Can you work these out from the model? Positions are in its coordinate system, mm. Face numbers are marked on the shaded views. A direction names the side the tool comes from. Round coordinates to 2 decimals unless told otherwise and drop trailing zeros. Order: outer loops, then holes, each group sorted by start corner. A loop starts at its lowest first (then second) coordinate and runs counter-clockwise, first axis right, second up. Notation, with made-up numbers: (3.5, -17) -> (28.5, -17) arc R28 ccw to (28.5, 10) -> close; hole circle Ø3 at (43.5, 49). An arc over 180 degrees is marked (long way). One line per item, written item: value.
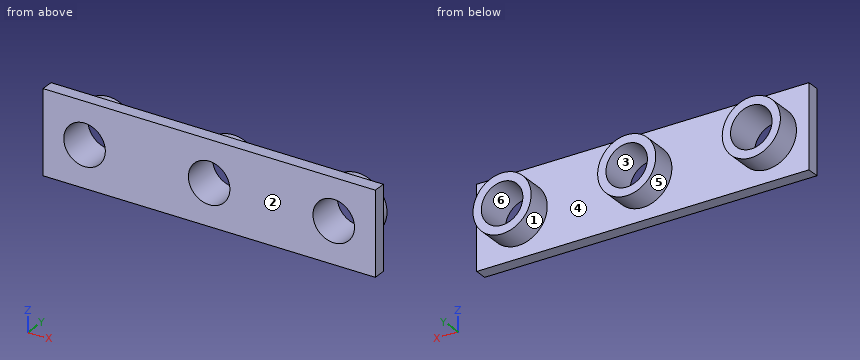
Autodesk Inventor part; units mm, degrees
ref_plane "YZ Plane" through (0, 0, 0) normal (1, 0, 0) x (0, 1, 0)
ref_plane "XZ Plane" through (0, 0, 0) normal (0, 1, 0) x (-1, 0, 0)
ref_plane "XY Plane" through (0, 0, 0) normal (0, 0, 1) x (1, 0, 0)
sketch "Sketch1" plane through (0, 0, 0) normal (0, 1, 0) x (-1, 0, 0)
  line L0 (20, -5) -> (-20, -5)
  line L1 (-20, -5) -> (-20, 5)
  line L2 (-20, 5) -> (20, 5)
  line L3 (20, 5) -> (20, -5)
  circle A0 centre (0, 0) radius 2.5
  line L4 (0, 0) -> (15, 0)
  circle A1 centre (15, 0) radius 2.5
  line L5 (0, 0) -> (-15, 0)
  circle A2 centre (-15, 0) radius 2.5
  dimension "d0" = 40
  dimension "d1" = 10
  dimension "d13" = 5
  dimension "d14" = 15
  dimension "d15" = 5
  dimension "d16" = 15
  dimension "d17" = 5
extrude "Extrusion1" add sketch "Sketch1" along normal blind 1.5
sketch "Sketch4" plane through (0, 1.5, 0) normal (0, 1, 0) x (1, 0, 0)
  circle A0 centre (0, 0) radius 3.5
  circle A1 centre (-15, 0) radius 3.5
  circle A2 centre (15, 0) radius 3.5
  circle A3 centre (-15, 0) radius 2.5
  circle A4 centre (0, 0) radius 2.5
  circle A5 centre (15, 0) radius 2.5
  dimension "d18" = 7
  dimension "d21" = 7
  dimension "d22" = 7
  dimension "d23" = 1
  dimension "d24" = 1
  dimension "d25" = 1
extrude "Extrusion3" add sketch "Sketch4" along normal blind 3
properties part number "GANJEL LED PLA"
Q1. I want a section at B-B on y = 0.45. List the corners of the cut face in (x, z) for me.
Answers below:
outline: (-20, -5) -> (20, -5) -> (20, 5) -> (-20, 5) -> close; hole circle Ø5 at (-15, 0); hole circle Ø5 at (0, 0); hole circle Ø5 at (15, 0)
Q2. On a 3-axis mill with a long thin cutter (end or side, diameter ignored), from which of +Z, -Z, +X, -X, +Y, -Y can I reach the whole of each face in a straight line? I mean the marked faces 1 and 2. Say none if no direction works.
Answers below:
face 1: +Y
face 2: +Z, -Z, +X, -X, -Y
Q3. Will these pins go through, and if not, where does the flat tip stop? pin 1 Ø2 at (y, z) = (3, 2) entering from +X; pin 2 Ø3 at (x, z) = (-15, 0) entering from -Y; pin 3 Ø2 at (y, z) = (3.5, 3) entering from -X.
Answers below:
pin 1: x = 18.35
pin 2: through
pin 3: x = -17.87
Q4. Please list where these lines run through material, in increasing order: line 1 along X through (y, z) = (2.3, 0); line 2 along Z through (x, y) = (15, 3.25); line 3 along Y through (x, z) = (10, -2.5).
Answers below:
line 1: -18.5 to -17.5, -12.5 to -11.5, -3.5 to -2.5, 2.5 to 3.5, 11.5 to 12.5, 17.5 to 18.5
line 2: -3.5 to -2.5, 2.5 to 3.5
line 3: 0 to 1.5
Q5. I want a section at C-C on z = -2. List the corners of the cut face in (x, y) for me, plus the area to 3 significant figures.
Answers below:
outline: (-20, 0) -> (-16.5, 0) -> (-16.5, 4.5) -> (-17.87, 4.5) -> (-17.87, 1.5) -> (-20, 1.5) -> close; (-13.5, 0) -> (-1.5, 0) -> (-1.5, 4.5) -> (-2.87, 4.5) -> (-2.87, 1.5) -> (-12.13, 1.5) -> (-12.13, 4.5) -> (-13.5, 4.5) -> close; (1.5, 0) -> (13.5, 0) -> (13.5, 4.5) -> (12.13, 4.5) -> (12.13, 1.5) -> (2.87, 1.5) -> (2.87, 4.5) -> (1.5, 4.5) -> close; (16.5, 0) -> (20, 0) -> (20, 1.5) -> (17.87, 1.5) -> (17.87, 4.5) -> (16.5, 4.5) -> close
area: 71.2 mm^2
Q6. We'd pull the mould along Z, two halves only. Please class the marked faces 3, 4, 5 and 6: released by +Z, released by -Z, zero draft, split by the parting line, or undercut.
Answers below:
face 3: undercut
face 4: zero draft
face 5: split by the parting line
face 6: undercut
Q7. I want a section at A-A on y = 2.25. List the corners of the cut face in (x, z) for me, plus the area to 3 significant figures.
Answers below:
outline: circle Ø7 at (-15, 0); circle Ø7 at (0, 0); circle Ø7 at (15, 0); hole circle Ø5 at (-15, 0); hole circle Ø5 at (0, 0); hole circle Ø5 at (15, 0)
area: 56.5 mm^2
